Input: part model. Units: mm. Frame: model coordinates. A direction names the side the tool comes from. Give positions to 0.01 mm unless a question says otherwise; leave off trailing zeros. Loops run counter-clockwise (first coordinate to the right, second up) from the corner with the lowest first, then second, coordinate; pieces in that order, holes last. Notation, with made-up numbers: (74.5, 51.5) -> (81.5, 51.5) arc R7 ccw to (81.5, 56.5) -> close; hole circle Ø11 at (88, -13). An arc over 180 degrees is marked (long way). Answer as a JSON object with one key per item and string values.
Autodesk Inventor part; units mm, degrees
ref_plane "Work Plane1" through (0, 0, 15) normal (0, 0, -1) x (-1, 0, 0)
ref_plane "YZ Plane" through (0, 0, 0) normal (1, 0, 0) x (0, 1, 0)
ref_plane "XZ Plane" through (0, 0, 0) normal (0, 1, 0) x (-1, 0, 0)
sketch "Sketch1" plane through (0, 0, 0) normal (0, 0, 1) x (1, 0, 0)
  line L0 (-6.075, -2.575) -> (6.075, -2.575)
  line L1 (6.075, -2.575) -> (6.075, 2.575)
  line L2 (6.075, 2.575) -> (-6.075, 2.575)
  line L3 (-6.075, 2.575) -> (-6.075, -2.575)
  line L4 (-6.075, -2.575) -> (6.075, 2.575) construction
  line L5 (6.075, -2.575) -> (-6.075, 2.575) construction
  line L6 (-8.075, 4.575) -> (8.075, 4.575)
  line L7 (8.075, 4.575) -> (8.075, -4.575)
  line L8 (8.075, -4.575) -> (-8.075, -4.575)
  line L9 (-8.075, -4.575) -> (-8.075, 4.575)
  point P0 (0, 0)
  dimension "d0" = 5.15
  dimension "d1" = 12.15
  dimension "d2" = 2
extrude "Extrusion1" add sketch "Sketch1" along normal blind 30
sketch "Sketch2" plane through (0, 0, 30) normal (0, 0, 1) x (1, 0, 0)
  line L0 (14.575, -11.075) -> (-14.575, -11.075)
  line L1 (-14.575, -11.075) -> (-14.575, 11.075)
  line L2 (-14.575, 11.075) -> (14.575, 11.075)
  line L3 (14.575, 11.075) -> (14.575, -11.075)
  line L4 (14.575, -11.075) -> (-14.575, 11.075) construction
  line L5 (-14.575, -11.075) -> (14.575, 11.075) construction
  line L6 (8.075, 4.575) -> (-8.075, 4.575) construction
  line L7 (-8.075, 4.575) -> (-8.075, -4.575) construction
  line L8 (8.075, -4.575) -> (8.075, 4.575) construction
  line L9 (-6.075, -2.575) -> (-6.075, 2.575)
  line L10 (-6.075, 2.575) -> (6.075, 2.575)
  line L11 (6.075, 2.575) -> (6.075, -2.575)
  line L12 (6.075, -2.575) -> (-6.075, -2.575)
  line L13 (8.075, 4.575) -> (-8.075, 4.575)
  line L14 (-8.075, 4.575) -> (-8.075, -4.575)
  line L15 (-8.075, -4.575) -> (8.075, -4.575) construction
  line L16 (8.075, -4.575) -> (8.075, 4.575)
  point P0 (0, 0)
  dimension "d5" = 6.5
  dimension "d6" = 6.5
extrude "Extrusion2" add sketch "Sketch2" along normal blind 1
ref_plane "Work Plane1" through (0, 0, 15) normal (0, 0, -1) x (-1, 0, 0)
mirror "Mirror1" about plane through (0, 0, 15) normal (0, 0, -1) of "Extrusion2"
fillet "Fillet1" radius 4 4 edges at (8.075, 4.575, 15) (8.075, -4.575, 15) (-8.075, -4.575, 15) (-8.075, 4.575, 15)
sketch "Sketch3" plane through (0, 0, 31) normal (0, 0, 1) x (1, 0, 0)
  line L0 (6.075, 2.575) -> (6.075, -2.575)
  line L1 (-6.075, 2.575) -> (6.075, 2.575)
  line L2 (-6.075, -2.575) -> (-6.075, 2.575)
  line L3 (6.075, -2.575) -> (-6.075, -2.575)
  line L4 (-6.975, -3.475) -> (-6.975, 3.475)
  line L5 (-6.975, 3.475) -> (6.975, 3.475)
  line L6 (6.975, 3.475) -> (6.975, -3.475)
  line L7 (6.975, -3.475) -> (-6.975, -3.475)
  point P0 (0, 0)
  dimension "d10" = 0.9
extrude "Extrusion3" add sketch "Sketch3" along normal blind 3.9
mirror "Mirror2" about plane through (0, 0, 15) normal (0, 0, -1) of "Extrusion3"
sketch "Sketch5" plane through (0, 0, 30) normal (0, 0, -1) x (-1, 0, 0)
  line L0 (-8.075, -0.575) -> (-8.075, 0.575) construction
  line L1 (-20.405, 0) -> (20.405, 0) construction
  line L2 (-8.075, -1.5) -> (-14.575, -1.5) construction
  line L3 (-14.575, -1.5) -> (-14.575, 1.5) construction
  line L4 (-14.575, 1.5) -> (-8.075, 1.5) construction
  line L5 (-8.075, 1.5) -> (-8.075, -1.5) construction
  line L6 (-8.075, -1.5) -> (-14.575, 1.5) construction
  line L7 (-14.575, -1.5) -> (-8.075, 1.5) construction
  line L8 (-14.575, -11.075) -> (-14.575, 11.075) construction
  arc A0 (-9.575, -1.5) -> (-9.575, 1.5) centre (-9.575, 0) ccw
  line L9 (-9.575, 1.5) -> (-14.575, 1.5)
  line L10 (-14.575, 1.5) -> (-14.575, -1.5)
  line L11 (-14.575, -1.5) -> (-9.575, -1.5)
  line L12 (-9.575, 0) -> (-9.575, 1.9655) construction
  line L13 (11.575, 3.0291) -> (11.575, -4.4188) construction
  line L14 (14.575, 11.075) -> (14.575, -11.075) construction
  line L15 (14.575, -1.5) -> (11.575, -1.5) construction
  line L16 (11.575, -1.5) -> (11.575, 1.5) construction
  line L17 (11.575, 1.5) -> (14.575, 1.5) construction
  line L18 (14.575, 1.5) -> (14.575, -1.5) construction
  line L19 (14.575, -1.5) -> (11.575, 1.5) construction
  line L20 (11.575, -1.5) -> (14.575, 1.5) construction
  arc A1 (13.075, 1.5) -> (13.075, -1.5) centre (13.075, 0) ccw
  line L21 (13.075, 1.5) -> (14.575, 1.5)
  line L22 (14.575, 1.5) -> (14.575, -1.5)
  line L23 (14.575, -1.5) -> (13.075, -1.5)
  point P0 (0, 0)
  point P1 (-11.325, 0)
  dimension "d13" = 3
  dimension "d14" = 1.5
  dimension "d15" = 3
  dimension "d16" = 1.5
  dimension "d17" = 3
extrude "Extrusion4" cut sketch "Sketch5" against normal through all
fillet "Fillet2" radius 0.5 12 edges at (14.575, 1.5, 30.5) (14.575, -1.5, 30.5) (-14.575, 1.5, 30.5) (-14.575, -1.5, 30.5) (-14.575, 11.075, 30.5) (14.575, 11.075, 30.5) (14.575, -11.075, 30.5) (-14.575, -11.075, 30.5) (-14.575, -11.075, -0.5) (-14.575, 11.075, -0.5) (14.575, 11.075, -0.5) (14.575, -11.075, -0.5)
equation "\"d2\" = ep"
equation "\"ep\" = 2"
properties part number "kicker_tube" material "Nylon 6/6"
Q1. Section D-D, the plane z = 5. Return the cut outline in (x, y) (3 decimals).
Evaluation:
{"outline": "(-8.075, -0.575) arc R4 ccw to (-4.075, -4.575) -> (4.075, -4.575) arc R4 ccw to (8.075, -0.575) -> (8.075, 0.575) arc R4 ccw to (4.075, 4.575) -> (-4.075, 4.575) arc R4 ccw to (-8.075, 0.575) -> close; hole (-6.075, -2.575) -> (6.075, -2.575) -> (6.075, 2.575) -> (-6.075, 2.575) -> close"}
Q2. Section B-B, the plane x = 12. Return the cut outline in (y, z) (3 decimals), then the cut area to 3 significant figures.
Evaluation:
{"outline": "(-11.075, -1) -> (11.075, -1) -> (11.075, 0) -> (-11.075, 0) -> close; (-11.075, 30) -> (-1.5, 30) -> (-1.5, 31) -> (-11.075, 31) -> close; (1.5, 30) -> (11.075, 30) -> (11.075, 31) -> (1.5, 31) -> close", "area": "41.3 mm2"}
Q3. Section C-C, the plane x = -1.25. Return the cut outline in (y, z) (3 decimals).
Evaluation:
{"outline": "(-11.075, -1) -> (-3.475, -1) -> (-3.475, -4.9) -> (-2.575, -4.9) -> (-2.575, 34.9) -> (-3.475, 34.9) -> (-3.475, 31) -> (-11.075, 31) -> (-11.075, 30) -> (-4.575, 30) -> (-4.575, 0) -> (-11.075, 0) -> close; (2.575, -4.9) -> (3.475, -4.9) -> (3.475, -1) -> (11.075, -1) -> (11.075, 0) -> (4.575, 0) -> (4.575, 30) -> (11.075, 30) -> (11.075, 31) -> (3.475, 31) -> (3.475, 34.9) -> (2.575, 34.9) -> close"}
Q4. Access query for faces 3 (the flat face through (0, -4.575, 15)), 4 (the flat face through (8.075, 0, 15)), 5 (the flat face through (-13.6, 1.5, 30.5)), 6 (the flat face through (-6.975, 0, -3)). Directions: +Z, -Z, +X, -X, +Y, -Y. A direction counts if a zero-diameter tool reaches every point of the face in a straight line with its end or side. Return the directions, or none.
Evaluation:
{"face 3": "+X, -X, -Y", "face 4": "+X, +Y, -Y", "face 5": "+Z, -X", "face 6": "-Z, -X, +Y, -Y"}
Q5. Pin query (flat end, axial travel): pin 1 (2.5 mm diameter, centred on y = 1, z = 22, fed in from +X) (3 decimals); pin 2 (9.5 mm diameter, centred on x = 3, z = 23.5, fed in from -Y) (3 decimals); pin 3 (2 mm diameter, centred on x = 0, y = -1.5, fed in from -Z); pin 4 (1.5 mm diameter, centred on y = -1, z = 11.5, fed in from -X) (3 decimals). Return the tip coordinate at first contact, or that it passes through.
Evaluation:
{"pin 1": "stops at x = 8.075", "pin 2": "stops at y = -4.575", "pin 3": "passes through", "pin 4": "stops at x = -8.075"}
Q6. Section A-A, the plane y = 8.25. Return the cut outline in (x, z) (3 decimals).
Evaluation:
{"outline": "(-14.575, -1) -> (14.575, -1) -> (14.575, 0) -> (-14.575, 0) -> close; (-14.575, 30) -> (14.575, 30) -> (14.575, 31) -> (-14.575, 31) -> close"}
Q7. Draft query along Z for faces 1 (the flat face through (0, 3.475, -3)), 2 (the flat face through (0, 4.575, 15)). Return one class per face: +Z half, -Z half, draft (parallel to the pull), parting line (faces both ways), or undercut.
Evaluation:
{"face 1": "draft", "face 2": "undercut"}
Q8. Ray query, line 1 along X through (y, z) = (1.25, 32) (3 decimals); line 2 along Z through (x, y) = (5.25, 5.5); line 3 along Y through (x, z) = (2, 22) (3 decimals). Return the intervals inside material, ascending.
Evaluation:
{"line 1": "x = -6.975 to -6.075, 6.075 to 6.975", "line 2": "z = -1 to 0, 30 to 31", "line 3": "y = -4.575 to -2.575, 2.575 to 4.575"}
